Input: dimensioned drawing with shaded views. Units: mm. Origin: part minimum x, y, z. A direction names the side the tool comes from. Round coordinates to 2 decimals unless told otherwise and drop trailing zeros. Loops run counter-clockwise (first coordinate to the right, second up) from the corner with the lowest first, then second, coordinate; pieces in that order, holes last.
1) Section D-D, the plane x = 105. Return loops of the section in (y, z).
2) Draft query along Y for the marked faces 6, 7 and 8. Return one class per face: pulls with the +Y half, pulls with the -Y half, needs draft (parallel to the pull), parting line crosses it, or undercut.
3) Section C-C, the plane y = 191.5. Return loops of the section in (x, z).
4) Section A-A, the plane z = 56. State how many separate pieces and enclosed holes the cut face has, and give its area (3 significant figures).
5) Ray query, line 1 along Y through (x, z) = (82.5, 92.5); line 2 along X through (y, z) = (164, 97); line 3 along Y through (x, z) = (147, 54). Return the intervals inside material, ascending.
6) Access query for the marked faces 1, 2, 3, 4 and 5. Directions: +Z, -Z, +X, -X, +Y, -Y. A direction counts if a zero-diameter tool reaches every point of the face in a straight line with its end or side. Return the directions, or none.
7) First-contact query: pin 1 (2.5 mm diameter, centred on y = 3.5, z = 31.5, fed in from +X) (1 decimal); pin 2 (1 mm diameter, centred on y = 113, z = 69.5, fed in from +X); pin 3 (10.5 mm diameter, centred on x = 133.5, z = 75, fed in from +Y). Flat tips, straight axial feed; report the tip coordinate or a pass-through.
8) Section B-B, the plane x = 134.2. Return loops of the section in (y, z), and give its area (3 significant figures).
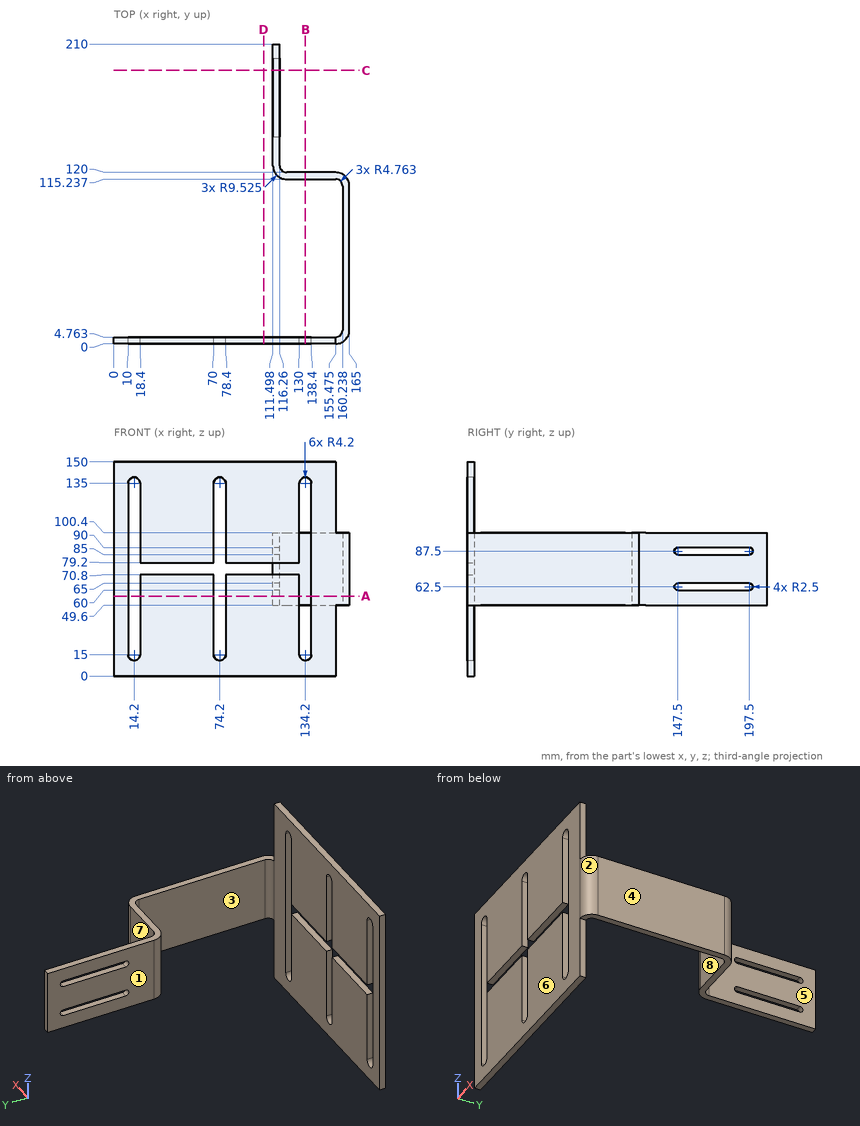
Final values:
1. outline: (0, 0) - (4.76, 0) - (4.76, 70.8) - (0, 70.8) - close; (0, 79.2) - (4.76, 79.2) - (4.76, 150) - (0, 150) - close
2. face 6: pulls with the -Y half
2. face 7: pulls with the +Y half
2. face 8: undercut
3. outline: (111.5, 49.6) - (116.26, 49.6) - (116.26, 60) - (111.5, 60) - close; (111.5, 65) - (116.26, 65) - (116.26, 85) - (111.5, 85) - close; (111.5, 90) - (116.26, 90) - (116.26, 100.4) - (111.5, 100.4) - close
4. separate pieces: 4
4. enclosed holes: 0
4. area: 1,830 mm2
5. line 1: y = 0 to 4.76
5. line 2: x = 111.5 to 116.26
5. line 3: y = 0 to 4.76, 115.24 to 120
6. face 1: +Z, -Z, -X, +Y
6. face 2: +Z, -Z, +X, -Y
6. face 3: +Z, -Z, -X
6. face 4: +Z, -Z, +X, +Y, -Y
6. face 5: +Z, -Z, +X, +Y
7. pin 1: stops at x = 155.5
7. pin 2: stops at x = 164.78
7. pin 3: stops at y = 120
8. outline: (0, 0) - (4.76, 0) - (4.76, 10.8) - (0, 10.8) - close; (0, 139.2) - (4.76, 139.2) - (4.76, 150) - (0, 150) - close; (115.24, 49.6) - (120, 49.6) - (120, 100.4) - (115.24, 100.4) - close
8. area: 345 mm2
